```python
from build123d import *

# Parameters (mm, degrees)
ESQUISSE2_R             = 14
ESQUISSE2_R_2           = 1.7
BOSS_EXTRU_1_DEPTH      = 5
BOSS_EXTRU_2_DEPTH      = 5
BOSS_EXTRU_3_DEPTH      = 20
CHANFREIN1_SIZE         = 20
ENL_V_MAT_EXTRU_1_DEPTH = 25
CHANFREIN2_SIZE         = 6
ESQUISSE6_R             = 2.65
ENL_V_MAT_EXTRU_2_DEPTH = 25
ESQUISSE7_R             = 2.65
ENL_V_MAT_EXTRU_3_DEPTH = 25


# Some blends are built 0.0001 mm under size
with BuildPart() as part:
    # Esquisse2 → Boss.-Extru.1 (new body)
    with BuildSketch(Plane.XY):
        with BuildLine():
            Line((12.489995997, 17.5), (-12.489995997, 17.5))
            ThreePointArc((-12.489995997, 17.5), (-15.202795796, 15.202795796), (-17.5, 12.489995997))
            Line((-17.5, 12.489995997), (-17.5, -12.489995997))
            ThreePointArc((-17.5, -12.489995997), (-15.202795796, -15.202795796), (-12.489995997, -17.5))
            Line((-12.489995997, -17.5), (12.489995997, -17.5))
            ThreePointArc((12.489995997, -17.5), (15.202795796, -15.202795796), (17.5, -12.489995997))
            Line((17.5, -12.489995997), (17.5, 12.489995997))
            ThreePointArc((17.5, 12.489995997), (15.202795796, 15.202795796), (12.489995997, 17.5))
        make_face()
        Circle(ESQUISSE2_R, mode=Mode.SUBTRACT)
        with Locations((-12.374368671, -12.374368671)):
            Circle(ESQUISSE2_R_2, mode=Mode.SUBTRACT)
        with Locations((12.374368671, -12.374368671)):
            Circle(ESQUISSE2_R_2, mode=Mode.SUBTRACT)
        with Locations((12.374368671, 12.374368671)):
            Circle(ESQUISSE2_R_2, mode=Mode.SUBTRACT)
        with Locations((-12.374368671, 12.374368671)):
            Circle(ESQUISSE2_R_2, mode=Mode.SUBTRACT)
    extrude(amount=BOSS_EXTRU_1_DEPTH)



with BuildPart() as body_2:
    # Esquisse3 → Boss.-Extru.2 (new body)
    with BuildSketch(Plane.XY.offset(5)):
        with BuildLine():
            Line((-17.5, -12.489995997), (-17.5, -34))
            Line((-17.5, -34), (34, -34))
            Line((34, -34), (34, 17.5))
            Line((34, 17.5), (12.489995997, 17.5))
            ThreePointArc((12.489995997, 17.5), (15.202795796, 15.202795796), (17.5, 12.489995997))
            Line((17.5, 12.489995997), (17.5, -12.489995997))
            ThreePointArc((17.5, -12.489995997), (15.202795796, -15.202795796), (12.489995997, -17.5))
            Line((12.489995997, -17.5), (-12.489995997, -17.5))
            ThreePointArc((-12.489995997, -17.5), (-15.202795796, -15.202795796), (-17.5, -12.489995997))
        make_face()
    extrude(amount=-BOSS_EXTRU_2_DEPTH)


with BuildPart() as part_1:
    add(part.part)

    add(body_2.part)  # Boss.-Extru.3 merges body 2
    # Esquisse4 → Boss.-Extru.3 (add)
    with BuildSketch(Plane(origin=(0, 0, 0), x_dir=(-1, 0, 0), z_dir=(0, 0, -1))):
        Polygon((-34, 17.5), (-34, -34), (17.65, -34), (17.5, -30), (-30, -30), (-30, 17.5), align=None)
    extrude(amount=BOSS_EXTRU_3_DEPTH)

    # Chanfrein1
    chanfrein1_edges = [part_1.edges().sort_by_distance(p)[0] for p in [
        (32, 17.5, -20),
        (-17.575, -32, -20),
    ]]
    chamfer(chanfrein1_edges, length=CHANFREIN1_SIZE - 0.0001)  # a hair under: the kernel refuses the full size

    # Esquisse5 → Enlèv. mat.-Extru.1 (cut)
    with BuildSketch(Plane.XY):
        Polygon((-17.5, -34), (-17.5, -30), (-17.65, -34), align=None)
    extrude(amount=-ENL_V_MAT_EXTRU_1_DEPTH, mode=Mode.SUBTRACT)

    # Chanfrein2
    # the kernel refuses this chamfer: 6 mm, written as the material it takes off along each edge
    with BuildSketch(Plane(origin=(-17.5, -34, 20.430097928), x_dir=(0.9996219169112969, -0.027495876610582164, 0), z_dir=(0, 0, -1))) as chanfrein2_piece_1:
        Polygon((CHANFREIN2_SIZE * 0.999621916911, -CHANFREIN2_SIZE * 0.0274958766106), (-CHANFREIN2_SIZE * 0.0274958766106, -CHANFREIN2_SIZE * 0.999621916911), (0, 0), align=None)
    extrude(amount=36.010190498, mode=Mode.SUBTRACT)
    with BuildSketch(Plane(origin=(34, 17.5, -15.430197928), x_dir=(-0.9996219169112969, 0.027495876610585633, 0), z_dir=(0, 0, 1))) as chanfrein2_piece_2:
        Polygon((CHANFREIN2_SIZE * 0.999621916911, CHANFREIN2_SIZE * 0.0274958766106), (-CHANFREIN2_SIZE * 0.0274958766106, CHANFREIN2_SIZE * 0.999621916911), (0, 0), align=None)
    extrude(amount=35.860295856, mode=Mode.SUBTRACT)

    # Esquisse6 → Enlèv. mat.-Extru.2 (cut)
    with BuildSketch(Plane.ZY.offset(-30)):
        with Locations((-9.34, -4)):
            Circle(ESQUISSE6_R)
        with Locations((-9.34, -24)):
            Circle(ESQUISSE6_R)
    extrude(amount=-ENL_V_MAT_EXTRU_2_DEPTH, mode=Mode.SUBTRACT)

    # Esquisse7 → Enlèv. mat.-Extru.3 (cut)
    with BuildSketch(Plane(origin=(0, -30, 0), x_dir=(1, 0, 0), z_dir=(0, 1, 0))):
        with Locations(Location((1, 9.34, 0), (0, 0, 180))):
            Circle(ESQUISSE7_R)
        with Locations(Location((21, 9.34, 0), (0, 0, 180))):
            Circle(ESQUISSE7_R)
    extrude(amount=-ENL_V_MAT_EXTRU_3_DEPTH, mode=Mode.SUBTRACT)


solid = part_1.part
```
Model file for the job. Use its own axes, mm. A direction names the side the tool comes from. Coordinates: 2 decimals unless noted, no trailing zeros. Write each loop counter-clockwise with the first axis right and the second up, starting at its lowest first coordinate (ties: lowest second). Pieces come first, ordered by that corner, then holes. Notation, with made-up numbers: (77.25, -2.75) - (104.25, -2.75) arc R17 ccw to (104.25, 9.25) - close; hole circle Ø11 at (89.5, 35). An arc over 180 degrees is marked (long way). Use a Markdown table: item, result. Add a question column.
Item 1: Drop flat-ended pins along their axis: pin 1 (2 mm diameter, centred on x = -0.5, z = -1.5, fed in from +Y); pin 2 (5.5 mm diameter, centred on x = -12.37, y = -12.37, fed in from -Z); pin 3 (4 mm diameter, centred on y = -2, z = -4.5, fed in from -X). Give the stop position or say it passes through.
Item 2: 3-axis set-ups, long thin cutter, end or side, ignore diameter. For faces 1 (the face through (16, -6, 0)), 2 (the face through (12, -34, -7)): which of +Z, -Z, +X, -X, +Y, -Y reach the whole face in a straight line?
Item 3: Band-saw the part on A-A, the plane y = 0. Write the cut outline in (x, z).
Item 4: Drill centre lines: line 1 along Y through (x, z) = (12, 4); line 2 along Z through (x, y) = (-1, -23); line 3 along Y through (x, z) = (11, -4.5). Where is each one in solid material? Low to high.
Item 5: Two-plate mould, pull along Y, no slides. Class faces 3 (the face through (-10.753, -11.864, 2.465)), 4 (the face through (7, 17.5, 3)), 5 (the face through (-17.5, -7, 3)): pulls with the +Y half, pulls with the -Y half, needs draft (parallel to the pull), parting line crosses it, or undercut.
Item 6: Band-saw the part on B-B, the plane x = 1. Write the cut outline in (y, z).
Item 7: Band-saw the part on D-D, the plane z = -3. Write the cut outline in (x, y).
Item 8: Band-saw the part on C-C, the plane z = -11.25. Write the cut outline in (x, y), and give its area (3 significant figures).
A:
| question | item | result |
|---|---|---|
| 1 | pin 1 | stops at y = -30 |
| 1 | pin 2 | stops at z = 0 |
| 1 | pin 3 | stops at x = 30 |
| 2 | face 1 | -Z, -X, +Y |
| 2 | face 2 | +Z, -Z, +X, -X, -Y |
| 3 | outline | (-17.5, 0) - (-14, 0) - (-14, 5) - (-17.5, 5) - close; (14, 0) - (30, 0) - (30, -17.5) - (34, -17.5) - (34, 5) - (14, 5) - close |
| 4 | line 1 | y = -34 to -14.03, -10.72 to -7.21, 7.21 to 10.72, 14.03 to 17.5 |
| 4 | line 2 | z = 0 to 5 |
| 4 | line 3 | y = -34 to -30 |
| 5 | face 3 | undercut |
| 5 | face 4 | pulls with the +Y half |
| 5 | face 5 | needs draft |
| 6 | outline | (-34, -18.64) - (-30, -18.49) - (-30, -11.99) - (-34, -11.99) - close; (-34, -6.69) - (-30, -6.69) - (-30, 0) - (-13.96, 0) - (-13.96, 5) - (-34, 5) - close; (13.96, 0) - (17.5, 0) - (17.5, 5) - (13.96, 5) - close |
| 7 | outline | (-14.53, -30.97) - (-11.5, -34) - (34, -34) - (34, 11.5) - (31, 14.5) - (30, 14.5) - (30, -30) - (-14.5, -30) - close |
| 8 | outline | (-6.39, -34) - (-0.84, -34) - (-0.84, -30) - (-6.24, -30) - close; (2.84, -34) - (19.16, -34) - (19.16, -30) - (2.84, -30) - close; (22.84, -34) - (34, -34) - (34, -25.84) - (30, -25.84) - (30, -30) - (22.84, -30) - close; (30, -22.16) - (34, -22.16) - (34, -5.84) - (30, -5.84) - close; (30, -2.16) - (34, -2.16) - (34, 6.25) - (30, 6.25) - close |
| 8 | area | 247 mm² |
